Model file for the job. Use its own axes, mm. Round coordinates to 2 decimals unless told otherwise and drop trailing zeros. Order: outer loops, then holes, each group sorted by start corner. A loop starts at its lowest first (then second) coordinate and runs counter-clockwise, first axis right, second up. Notation, with made-up numbers: (5.5, -37) - (57.5, -37) arc R13 ccw to (57.5, -12) - close; hole circle Ø5 at (62, -39). An arc over 180 degrees is marked (long way). Write item = value, one per line.
```python
from build123d import *

# Parameters (mm, degrees)
SKETCH1_R                  = 5.5
SKETCH1_R_2                = 4.5
BOSS_EXTRUDE1_DEPTH        = 67.5
IZIM2_R                    = 1
KES_EKSTR_ZYON1_DEPTH      = 6.5
KES_EKSTR_ZYON1_DEPTH_BACK = 6.5
IZIM3_R                    = 1
KES_EKSTR_ZYON2_DEPTH      = 6.500000118
KES_EKSTR_ZYON2_DEPTH_BACK = 6.500000118


with BuildPart() as part:
    # Sketch1 → Boss-Extrude1 (new body)
    with BuildSketch(Plane.XY):
        Circle(SKETCH1_R)
        Circle(SKETCH1_R_2, mode=Mode.SUBTRACT)
    extrude(amount=BOSS_EXTRUDE1_DEPTH)

    # Çizim2 → Kes-Ekstrüzyon1 (cut, two sides)
    with BuildSketch(Plane(origin=(0, 0, 0), x_dir=(1, 0, 0), z_dir=(0, 1, 0))) as kes_ekstr_zyon1_sk:
        with Locations((0, -7)):
            Circle(IZIM2_R)
    extrude(amount=KES_EKSTR_ZYON1_DEPTH, mode=Mode.SUBTRACT)
    extrude(kes_ekstr_zyon1_sk.sketch, amount=-KES_EKSTR_ZYON1_DEPTH_BACK, mode=Mode.SUBTRACT)

    # Çizim3 → Kes-Ekstrüzyon2 (cut, two sides)
    with BuildSketch(Plane(origin=(0, 0, 0), x_dir=(1, 0, 0), z_dir=(0, 1, 0))) as kes_ekstr_zyon2_sk:
        with Locations((0, -62.5)):
            Circle(IZIM3_R)
    extrude(amount=KES_EKSTR_ZYON2_DEPTH, mode=Mode.SUBTRACT)
    extrude(kes_ekstr_zyon2_sk.sketch, amount=-KES_EKSTR_ZYON2_DEPTH_BACK, mode=Mode.SUBTRACT)


solid = part.part
```
1) Cut at C-C (x = -3.75). Write the cut outline in (y, z), and give its area (3 significant figures).
Conclusion:
outline = (-4.02, 0) - (-2.49, 0) - (-2.49, 67.5) - (-4.02, 67.5) - close; (2.49, 0) - (4.02, 0) - (4.02, 67.5) - (2.49, 67.5) - close
area = 207 mm^2
2) Wall check: line 1 along Z through (x, y) = (0, 5); line 2 along Y through (x, z) = (0, 52); line 3 along Y through (x, z) = (-1.5, 37.5). Give the ranges that are in metal, low to high.
Conclusion:
line_1 = 0 to 6, 8 to 61.5, 63.5 to 67.5
line_2 = -5.5 to -4.5, 4.5 to 5.5
line_3 = -5.29 to -4.24, 4.24 to 5.29
3) Cut at D-D (z = 56.5). Write the cut outline in (x, y), and give its area (3 significant figures).
Conclusion:
outline = circle Ø11 at (0, 0); hole circle Ø9 at (0, 0)
area = 31.4 mm^2
4) Cut at A-A (x = 0). Write the cut outline in (y, z), and give its area (3 significant figures).
Conclusion:
outline = (-5.5, 0) - (-4.5, 0) - (-4.5, 6) - (-5.5, 6) - close; (-5.5, 8) - (-4.5, 8) - (-4.5, 61.5) - (-5.5, 61.5) - close; (-5.5, 63.5) - (-4.5, 63.5) - (-4.5, 67.5) - (-5.5, 67.5) - close; (4.5, 0) - (5.5, 0) - (5.5, 6) - (4.5, 6) - close; (4.5, 8) - (5.5, 8) - (5.5, 61.5) - (4.5, 61.5) - close; (4.5, 63.5) - (5.5, 63.5) - (5.5, 67.5) - (4.5, 67.5) - close
area = 127 mm^2
5) Flat gauge pins, fed straight in: pin 1 Ø3 at (y, z) = (-2.5, 40) entering from +X; pin 2 Ø2 at (x, z) = (2, 10) entering from +Y; pin 3 Ø1 at (x, z) = (2, 41) entering from +Y. Where does each tip first touch, or does it go through?
Conclusion:
pin_1 = 5.41
pin_2 = 5.41
pin_3 = 5.29
6) Mould opens along X. For faces 1 (the face through (-1.19, -5.37, 33.28)), 2 (the face through (-5, 0, 67.5)), 3 (the face through (-0.8, 4.9, 7.6)) say: +X half, -X half, draft (parallel to the pull), parting line (faces both ways), or undercut.
Conclusion:
face_1 = parting line
face_2 = draft
face_3 = undercut
7) Cut at B-B (y = 0). Write the cut outline in (x, z), and give its area (3 significant figures).
Conclusion:
outline = (-5.5, 0) - (-4.5, 0) - (-4.5, 67.5) - (-5.5, 67.5) - close; (4.5, 0) - (5.5, 0) - (5.5, 67.5) - (4.5, 67.5) - close
area = 135 mm^2
